```python
from build123d import *

# Parameters (mm, degrees)
BOSS_EXTRUDE1_DEPTH = 13.462
SKETCH7_OUTSIDE_W   = 29.274
SKETCH7_OUTSIDE_H   = 34.1
SKETCH7_OUTSIDE_R   = 13.462
CUT_EXTRUDE1_DEPTH  = 13.462
SKETCH8_R           = 1.524
CUT_EXTRUDE2_DEPTH  = 6.35
SKETCH9_R           = 6.35
CUT_EXTRUDE3_DEPTH  = 42.402
SKETCH10_R          = 0.381
CUT_EXTRUDE4_DEPTH  = 35.56
CIRPATTERN1_COUNT   = 8


with BuildPart() as part:
    # Sketch1 → Revolve1 (revolve)
    with BuildSketch(Plane.XY):
        Polygon((20.701, 0), (20.701, 8.636), (-17.653, 8.636), (-17.653, 7.112), (-19.431, 7.112), (-19.431, 8.636), (-20.701, 8.636), (-20.701, 0), align=None)
    revolve(axis=Axis((-78.241804248, 0, 0), (1, 0, 0)))

    # Sketch6 → Boss-Extrude1 (add)
    with BuildSketch(Plane(origin=(0, 0, 0), x_dir=(1, 0, 0), z_dir=(0, 1, 0))):
        Polygon((20.701, 0), (20.701, 4.699), (10.795, 4.699), (10.795, -4.699), (20.701, -4.699), align=None)
    extrude(amount=BOSS_EXTRUDE1_DEPTH)

    # Sketch7 outside → Cut-Extrude1 (cut)
    with BuildSketch(Plane(origin=(20.701, 0, 0), x_dir=(0, 0, -1), z_dir=(1, 0, 0))):
        with Locations((0, 2.413)):
            Rectangle(SKETCH7_OUTSIDE_W, SKETCH7_OUTSIDE_H)
        Circle(SKETCH7_OUTSIDE_R, mode=Mode.SUBTRACT)
    extrude(amount=-CUT_EXTRUDE1_DEPTH, mode=Mode.SUBTRACT)

    # Sketch8 → Cut-Extrude2 (cut)
    with BuildSketch(Plane(origin=(0, 13.462, 0), x_dir=(-1, 0, 0), z_dir=(0, 1, 0))):
        with Locations((-16.129, 0)):
            Circle(SKETCH8_R)
    extrude(amount=-CUT_EXTRUDE2_DEPTH, mode=Mode.SUBTRACT)

    # Sketch9 → Cut-Extrude3 (cut, through all)
    with BuildSketch(Plane(origin=(20.701, 0, 0), x_dir=(0, 0, -1), z_dir=(1, 0, 0))):
        Circle(SKETCH9_R)
    extrude(amount=-CUT_EXTRUDE3_DEPTH, mode=Mode.SUBTRACT)

    # Sketch10 → Cut-Extrude4 (cut)
    with BuildSketch(Plane(origin=(20.701, 0, 0), x_dir=(0, 0, -1), z_dir=(1, 0, 0))):
        with Locations((-5.916324211, 6.291073345)):
            Circle(SKETCH10_R)
    cut_extrude4 = extrude(amount=-CUT_EXTRUDE4_DEPTH, mode=Mode.SUBTRACT)

    # CirPattern1: Cut-Extrude4 ×8 about axis, 1 skipped
    cirpattern1_axis = Axis((20.701, 0, 0), (-1, 0, 0))
    add([cut_extrude4.rotate(cirpattern1_axis, i * 360 / CIRPATTERN1_COUNT) for i in range(1, CIRPATTERN1_COUNT) if i not in (1,)], mode=Mode.SUBTRACT)


solid = part.part
```
The model under review builds one solid part; all positions refer to its coordinate system, in mm. A direction names the side the tool comes from. Coordinates: 2 decimals unless noted, no trailing zeros. Write each loop counter-clockwise with the first axis right and the second up, starting at its lowest first coordinate (ties: lowest second). Pieces come first, ordered by that corner, then holes. Notation, with made-up numbers: (-14, 88) - (13, 88) arc R24 ccw to (13, 124) - close; hole circle Ø11 at (76.25, 19). An arc over 180 degrees is marked (long way). Answer in a Markdown table with one row per item. Add a question column.
Q1. Consider section A-A on y = 7.75. Give the boundary of the cut face in (x, z) (3 decimals), then the cut area to 3 significant figures.
Q2. To check wall thickness, follow line 1 along X through (y, z) = (8.75, 0) (3 decimals); line 2 along X through (y, z) = (-7.5, -3); line 3 along Y through (x, z) = (2, 0). State the ranges of each line that lie inside material, in increasing order. Write a range as from..to.
Q3. Draft analysis for pull direction Z (two halves, no side actions). For faces 4 (the face through (-19.431, -2, 7)), 5 (the face through (1.26, 8.24, 2.59)), 6 (the face through (16, 7.112, 0)), 7 (the face through (0.29, -6.2, 1.38)), state which applies: +Z half, -Z half, draft (parallel to the pull), parting line (faces both ways), or undercut.
Q4. Consider section C-C on y = -2.25. Give the boundary of the cut face in (x, z), then the cut area to 3 significant figures.
Q5. For faces 1 (the face through (14.675, 10.332, 0.458)), 2 (the face through (-18.554, -1.542, -6.943)), 3 (the face through (-20.075, -1.124, 8.563)), list the 3-axis set-ups (+Z, -Z, +X, -X, +Y, -Y) from which the entire face can be reached by the end or side of a thin tool; tool diameter is ignored.
Q6. Consider section D-D on x = 5. Give the boundary of the cut face in (y, z), then the cut area to 3 significant figures.
Q7. Clearance check with flat-ended pins moving along their axes: pin 1 (12 mm diameter, centred on x = -8.5, y = -6, fed in from -Z); pin 2 (5 mm diameter, centred on x = -4.5, z = 6.5, fed in from +Y); pin 3 (0.5 mm diameter, centred on y = -6, z = 6.5, fed in from +X). State where each tip first meets the part, or that it passes through.
Q8. Consider section B-B on z = -2.5. Give the boundary of the cut face in (x, y) (3 decimals).
Answers below:
| question | item | result |
|---|---|---|
| 1 | outline | (-20.701, -3.81) - (-19.431, -3.81) - (-19.431, 3.81) - (-20.701, 3.81) - close; (-17.653, -3.81) - (10.795, -3.81) - (10.795, -4.699) - (20.701, -4.699) - (20.701, 4.699) - (10.795, 4.699) - (10.795, 3.81) - (-17.653, 3.81) - close; hole circle Ø3.048 at (16.129, 0) |
| 1 | area | 312 mm² |
| 2 | line 1 | 10.795..14.605, 17.653..20.701 |
| 2 | line 2 | -20.7..-19.43, -17.65..20.7 |
| 2 | line 3 | -8.36..-6.35, 6.35..8.64 |
| 3 | face 4 | draft |
| 3 | face 5 | parting line |
| 3 | face 6 | undercut |
| 3 | face 7 | undercut |
| 4 | outline | (-20.7, -8.34) - (-19.43, -8.34) - (-19.43, -6.75) - (-17.65, -6.75) - (-17.65, -8.34) - (20.7, -8.34) - (20.7, -5.94) - (-20.7, -5.94) - close; (-20.7, 5.94) - (20.7, 5.94) - (20.7, 8.34) - (-17.65, 8.34) - (-17.65, 6.75) - (-19.43, 6.75) - (-19.43, 8.34) - (-20.7, 8.34) - close |
| 4 | area | 193 mm² |
| 5 | face 1 | +Y |
| 5 | face 2 | none |
| 5 | face 3 | -X |
| 6 | outline | (-8.64, -0.12) arc R8.64 ccw to (-6.55, -5.63) arc R0.38 cw to (-6.02, -6.19) arc R8.64 ccw to (-0.65, -8.61) arc R0.38 cw to (0.12, -8.64) arc R8.64 ccw to (5.63, -6.55) arc R0.38 cw to (6.19, -6.02) arc R8.64 ccw to (6.55, 5.63) arc R0.38 cw to (6.02, 6.19) arc R8.64 ccw to (0.65, 8.61) arc R0.38 cw to (-0.12, 8.64) arc R8.64 ccw to (-5.63, 6.55) arc R0.38 cw to (-6.19, 6.02) arc R8.64 ccw to (-8.61, 0.65) arc R0.38 cw to start; hole circle Ø12.7 at (0, 0) |
| 6 | area | 106 mm² |
| 7 | pin 1 | z = -8.61 |
| 7 | pin 2 | y = 7.65 |
| 7 | pin 3 | x = -14.86 |
| 8 | outline | (-20.701, -8.266) - (-19.431, -8.266) - (-19.431, -6.658) - (-17.653, -6.658) - (-17.653, -8.266) - (20.701, -8.266) - (20.701, -5.837) - (-20.701, -5.837) - close; (-20.701, 5.837) - (20.701, 5.837) - (20.701, 13.228) - (10.795, 13.228) - (10.795, 8.266) - (-17.653, 8.266) - (-17.653, 6.658) - (-19.431, 6.658) - (-19.431, 8.266) - (-20.701, 8.266) - close |
